Source: CAD feature listing. Evaluate the final solid. Frame: model axes, mm. A direction names the side the tool comes from. Give positions to 0.01 mm unless a question says otherwise; leave off trailing zeros. Order: outer loops, then holes, each group sorted by start corner. A loop starts at its lowest first (then second) coordinate and runs counter-clockwise, first axis right, second up. Notation, with made-up numbers: M -20.75,84.25 L 21.25,84.25 A20 ccw 21.25,119.25 Z; hole C 56,-15.5 d6. An arc over 180 degrees is marked long. Use CSV: the item, a comma, the result in double quotes. Start each with the question number.
Item 1: Ray query, probe 1 along Y at (x, z) = (-2, 3.5); probe 2 along X at (y, z) = (-4, 7); probe 3 along X at (y, z) = (0.5, 21). Return the intervals inside material, ascending. Write a range as from..to.
Item 2: Access query for faces 5 (the face through (57.15, 0, 13)), 6 (the face through (38.1, 0, 6)), 7 (the face through (-65.289, -3.414, 18.054)). Directions: +Z, -Z, +X, -X, +Y, -Y. A direction counts if a zero-diameter tool reaches every point of the face in a straight line with its end or side. Return the directions, or none.
Item 3: Section query A-A on z = 4.5. Return loops of the section in (x, y).
Item 4: Pull-direction query (Y, two-part tool) for faces 1 (the face through (-57.15, 4, 18)), 2 (the face through (-1, -19.05, 13)), 3 (the face through (-1, -6.35, 3)), 4 (the face through (-1, 6.35, 3)); classes: +Y half, -Y half, draft (parallel to the pull), parting line (faces both ways), or undercut.
Item 5: Section query D-D on z = 23.5. Return loops of the section in (x, y), and give its area (3 significant figures).
Item 6: First-contact query: pin 1 (6 mm diameter, centred on x = 23, y = 15, fed in from -Z); pin 2 (5 mm diameter, centred on x = 22.5, y = -1.5, fed in from -Z); pin 3 (1.5 mm diameter, centred on x = -25.5, y = 1.5, fed in from -Z); pin 4 (4 mm diameter, centred on y = 0, z = 5, fed in from -X). Flat tips, straight axial feed; report the tip coordinate or a pass-through.
from build123d import *

# Parameters (mm, degrees)
F0_W     = 114.3
F0_H     = 38.1
F1_DEPTH = 25.4
F2_R     = 6.35
F3_DEPTH = 19.05
F4_R     = 2.54
F5_W     = 101.6
F5_H     = 25.4
F6_DEPTH = 5.08
F7_SIZE  = 5.07999
F8_W     = 76.2
F8_H     = 12.7
F9_DEPTH = 12.7
F10_R    = 6.34999


# Not quite as in the source:
# - a fillet or chamfer is up to 0.001 mm smaller than in the source, because OpenCascade refuses the exact size


with BuildPart() as f1:
    # F0 (on Top) → F1 (new body)
    with BuildSketch(Plane.XY):
        Rectangle(F0_W, F0_H)
    extrude(amount=F1_DEPTH)

    # F2 (on face) → F3 (join)
    with BuildSketch(Plane(origin=(-57.15, 0, 0), x_dir=(0, -1, 0), z_dir=(-1, 0, 0))):
        with Locations((0, 12.7)):
            Circle(F2_R)
    extrude(amount=F3_DEPTH)

    # F4
    f4_edges = [f1.edges().sort_by_distance(p)[0] for p in [
        (-76.2, 6.35, 12.7),
    ]]
    fillet(f4_edges, radius=F4_R)

    # F5 (on face) → F6 (join)
    with BuildSketch(Plane.XY.offset(25.4)):
        Rectangle(F5_W, F5_H)
    extrude(amount=F6_DEPTH)

    # F7 (size 5.08 in the source; OpenCascade refuses exactly that, so slightly less here)
    f7_edges = [f1.edges().sort_by_distance(p)[0] for p in [
        (0, -12.7, 30.48),
        (-50.8, 0, 30.48),
        (50.8, 0, 30.48),
        (0, 12.7, 30.48),
    ]]
    chamfer(f7_edges, length=F7_SIZE)

    # F8 (on face) → F9 (cut)
    with BuildSketch(Plane(origin=(0, 0, 0), x_dir=(1, 0, 0), z_dir=(0, 0, -1))):
        Rectangle(F8_W, F8_H)
    extrude(amount=-F9_DEPTH, mode=Mode.SUBTRACT)

    # F10 (radius 6.35 in the source; OpenCascade refuses exactly that, so slightly less here)
    f10_edges = [f1.edges().sort_by_distance(p)[0] for p in [
        (0, 6.35, 12.7),
        (0, -6.35, 12.7),
    ]]
    fillet(f10_edges, radius=F10_R)


solid = f1.part
Verdict:
1,probe 1,"-19.05..-6.35, 6.35..19.05"
1,probe 2,"-57.15..-38.1, 38.1..57.15"
1,probe 3,"-57.15..57.15"
2,face 5,"+Z, -Z, +X, +Y, -Y"
2,face 6,"-Z"
2,face 7,"-X"
3,outline,"M -57.15,-19.05 L 57.15,-19.05 L 57.15,19.05 L -57.15,19.05 Z; hole M -38.1,-6.35 L 38.1,-6.35 L 38.1,6.35 L -38.1,6.35 Z"
4,face 1,"draft"
4,face 2,"-Y half"
4,face 3,"undercut"
4,face 4,"undercut"
5,outline,"M -57.15,-19.05 L 57.15,-19.05 L 57.15,19.05 L -57.15,19.05 Z"
5,area,"4,350 mm2"
6,pin 1,"z = 0"
6,pin 2,"z = 11.28"
6,pin 3,"z = 12.29"
6,pin 4,"x = -75.36"
